Verification items for the finished model (mm, model axes). A direction names the side the tool comes from. Give positions to 0.01 mm unless a question says otherwise; leave off trailing zeros. Write each loop counter-clockwise with the first axis right and the second up, starting at its lowest first coordinate (ties: lowest second). Pieces come first, ordered by that corner, then holes. Notation, with made-up numbers: (-2.5, -19) - (8.5, -19) arc R12 cw to (8.5, -5) - close; hole circle Ø8 at (-7.75, 24.25). An arc over 180 degrees is marked (long way). Put each result on its own line as item: value.
from build123d import *

# Parameters (mm, degrees)
FILLET_1_R = 4
FILLET_2_R = 2


with BuildPart() as part:
    # 草图1 → 旋转1 (revolve)
    with BuildSketch(Plane.XY, mode=Mode.PRIVATE) as revolve_1_sk:
        Polygon((-50, -14), (-50, 14), (-35, 14), (-35, 8), (-15, 8), (-15, 14), (-7, 14), (-7, -14), (-15, -14), (-15, -8), (-35, -8), (-35, -14), align=None)
    revolve(revolve_1_sk.sketch.rotate(Axis((0, 0, 0), (0, 1, 0)), 270), axis=Axis((0, 0, 0), (0, 1, 0)))

    # 圆角1
    fillet_1_edges = [part.edges().sort_by_distance(p)[0] for p in [
        (0, 14, 50),
        (0, -14, 50),
    ]]
    fillet(fillet_1_edges, radius=FILLET_1_R)

    # 圆角2
    fillet_2_edges = [part.edges().sort_by_distance(p)[0] for p in [
        (0, 8, 35),
    ]]
    fillet(fillet_2_edges, radius=FILLET_2_R)


solid = part.part
Q1. Release check for a two-part mould opening along Z. For faces 1 (the face through (6.834, -0.196, 1.517)), 2 (the face through (-15.02, 0.14, -47.69)), 3 (the face through (6.5, -14, 3.1)) record: released by +Z, released by -Z, zero draft, split by the parting line, or undercut.
Answers follow:
face 1: undercut
face 2: split by the parting line
face 3: zero draft
Q2. Go/stop test with flat-tipped pins: pin 1 Ø5 at (y, z) = (2, 23.5) entering from +X; pin 2 Ø8 at (y, z) = (-9, -30.5) entering from -X; pin 3 Ø3 at (x, y) = (-8, 6) entering from -Z. Record where each tip stops, or that it passes through.
Answers follow:
pin 1: stops at x = 45.38
pin 2: stops at x = -42.4
pin 3: stops at z = -49.58
Q3. Scan lines: line 1 along X through (y, z) = (-9.7, 0); line 2 along X through (y, z) = (-12.3, 0); line 3 along X through (y, z) = (-8.25, 8). Record each from-to range of solid material in increasing order.
Answers follow:
line 1: x = -50 to -35, -15 to -7, 7 to 15, 35 to 50
line 2: x = -49.27 to -35, -15 to -7, 7 to 15, 35 to 49.27
line 3: x = -49.36 to -34.07, -12.69 to 12.69, 34.07 to 49.36
Q4. Section check D-D, the plane y = -11.5. Record the cut outline in (x, z).
Answers follow:
outline: circle Ø99.42 at (0, 0); circle Ø30 at (0, 0); hole circle Ø70 at (0, 0); hole circle Ø14 at (0, 0)
Q5. Set-up check for faces 4 (the face through (-0.66, -10.958, 14.985)), 5 (the face through (14, 8, -7)), 6 (the face through (-31, -14, -17)): record each of +Z, -Z, +X, -X, +Y, -Y from which the full face is reachable in a straight line by a thin tool's end or side.
Answers follow:
face 4: -Y
face 5: +Y
face 6: +Z, -Z, +X, -X, -Y
Q6. Section check C-C, the plane y = -2.5. Record the cut outline in (x, z), plus the area to 3 significant figures.
Answers follow:
outline: circle Ø100 at (0, 0); hole circle Ø14 at (0, 0)
area: 7,700 mm2
